Input: dimensioned drawing with shaded views. Units: mm. Origin: part minimum x, y, z. Give positions to 0.01 mm unless a question says otherwise; leave off trailing zeros. Loops run counter-clockwise (first coordinate to the right, second up) from the corner with the lowest first, then second, coordinate; pieces in that order, holes last.
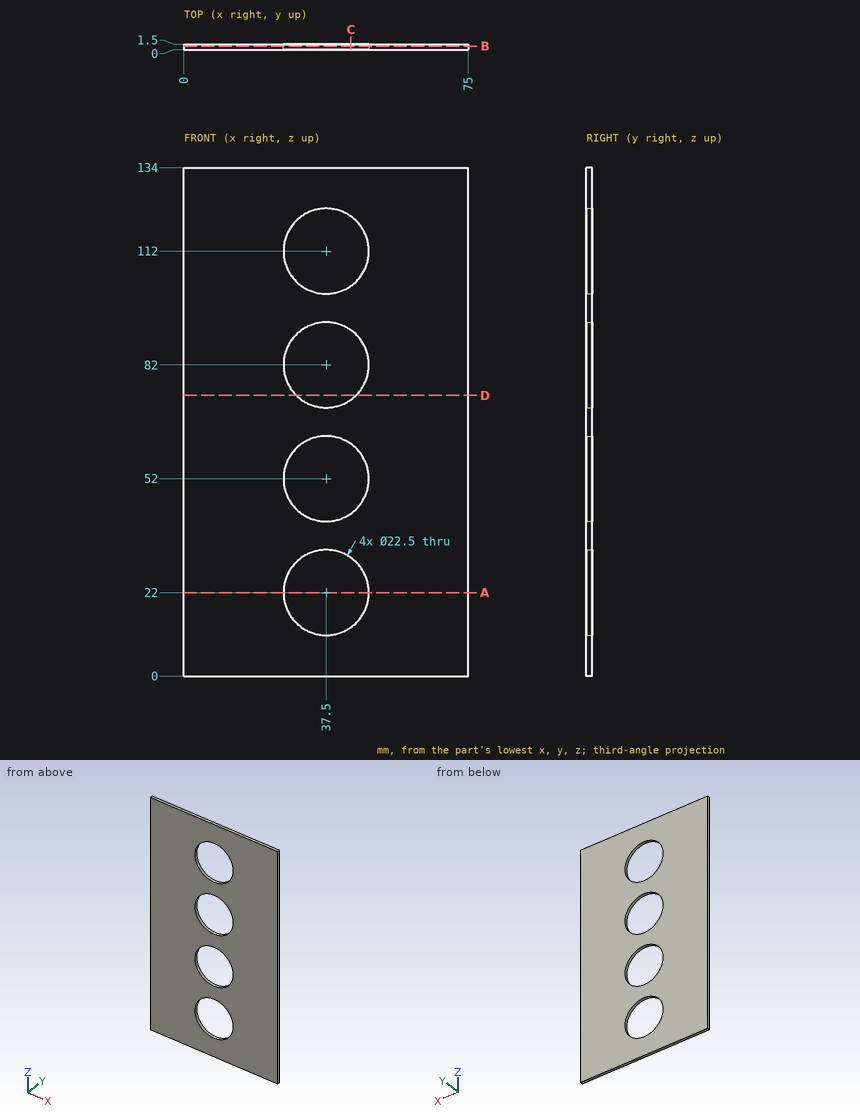
Item 1: Section query B-B on y = 0.95. Return loops of the section in (x, z), plus the area to 3 significant figures.
Values follow:
outline: (0, 0) - (75, 0) - (75, 134) - (0, 134) - close; hole circle Ø22.5 at (37.5, 22); hole circle Ø22.5 at (37.5, 52); hole circle Ø22.5 at (37.5, 82); hole circle Ø22.5 at (37.5, 112)
area: 8,460 mm2
Item 2: Section query C-C on x = 44. Return loops of the section in (y, z), plus the area to 3 significant figures.
Values follow:
outline: (0, 0) - (1.5, 0) - (1.5, 12.82) - (0, 12.82) - close; (0, 31.18) - (1.5, 31.18) - (1.5, 42.82) - (0, 42.82) - close; (0, 61.18) - (1.5, 61.18) - (1.5, 72.82) - (0, 72.82) - close; (0, 91.18) - (1.5, 91.18) - (1.5, 102.82) - (0, 102.82) - close; (0, 121.18) - (1.5, 121.18) - (1.5, 134) - (0, 134) - close
area: 90.8 mm2
Item 3: Pin query (flat end, axial travel): pin 1 (4 mm diameter, centred on x = 38.5, z = 39, fed in from -Y); pin 2 (13.5 mm diameter, centred on x = 37.5, z = 22, fed in from -Y). Return the tip coordinate at first contact, or that it passes through.
Values follow:
pin 1: stops at y = 0
pin 2: passes through
Item 4: Section query A-A on z = 22. Return loops of the section in (x, y), plus the area to 4 significant figures.
Values follow:
outline: (0, 0) - (26.25, 0) - (26.25, 1.5) - (0, 1.5) - close; (48.75, 0) - (75, 0) - (75, 1.5) - (48.75, 1.5) - close
area: 78.75 mm2
Item 5: Ray query, probe 1 along Z at (x, y) = (37.5, 0.85); probe 2 along Z at (x, y) = (41, 0.55); probe 3 along X at (y, z) = (1.2, 60.5). Return the intervals inside material, ascending.
Values follow:
probe 1: z = 0 to 10.75, 33.25 to 40.75, 63.25 to 70.75, 93.25 to 100.75, 123.25 to 134
probe 2: z = 0 to 11.31, 32.69 to 41.31, 62.69 to 71.31, 92.69 to 101.31, 122.69 to 134
probe 3: x = 0 to 30.13, 44.87 to 75
Item 6: Section query D-D on z = 74. Return loops of the section in (x, y), plus the area to 3 significant figures.
Values follow:
outline: (0, 0) - (29.59, 0) - (29.59, 1.5) - (0, 1.5) - close; (45.41, 0) - (75, 0) - (75, 1.5) - (45.41, 1.5) - close
area: 88.8 mm2
